from build123d import *

# Parameters (mm, degrees)
BOSS_EXTRUDE3_DEPTH = 4.5
SKETCH2_R           = 3.5
CUT_EXTRUDE2_DEPTH  = 4.5
SKETCH3_R           = 3.5
CUT_EXTRUDE3_DEPTH  = 4.5
SKETCH4_R           = 3.5
CUT_EXTRUDE4_DEPTH  = 4.5
SKETCH5_R           = 3.5
CUT_EXTRUDE5_DEPTH  = 4.5
SKETCH6_R           = 3.5
CUT_EXTRUDE6_DEPTH  = 4.5
SKETCH7_R           = 3.5
CUT_EXTRUDE7_DEPTH  = 4.5
SKETCH8_R           = 3.5
CUT_EXTRUDE8_DEPTH  = 4.5
SKETCH9_R           = 3.5
CUT_EXTRUDE9_DEPTH  = 4.5


with BuildPart() as part:
    # Sketch1 → Boss-Extrude3 (new body)
    with BuildSketch(Plane(origin=(0, 0, 0), x_dir=(1, 0, 0), z_dir=(0, 1, 0))):
        Polygon((-183.349573846, -2.857581752), (-179.118755434, 0), (-187.675629618, 0), align=None)
        Polygon((-179.118755434, 0), (-151.388696713, 0), (-165.408042798, 9.260497243), align=None)
        Polygon((-165.284400003, -14.790555769), (-147.342868955, -2.672476774), (-151.388696713, 0), (-179.118755434, 0), (-183.349573846, -2.857581752), align=None)
        Polygon((-147.342868955, -2.672476774), (-143.386109387, 0), (-151.388696713, 0), align=None)
        Polygon((-143.386109387, 0), (0, 96.845926684), (-35.732646047, 96.845926684), (-165.408042798, 9.260497243), (-151.388696713, 0), align=None)
        Polygon((-36.286932906, -100), (0, -100), (-147.342868955, -2.672476774), (-165.284400003, -14.790555769), align=None)
        Polygon((-165.408042798, 9.260497243), (-298.002482939, 96.845926684), (-319.003928208, 86.749077997), (-187.675629618, 0), (-179.118755434, 0), align=None)
        Polygon((-312.316233719, -89.964315732), (-291.442010442, -100), (-165.284400003, -14.790555769), (-183.349573846, -2.857581752), align=None)
        Polygon((0, -120), (0, -100), (-36.286932906, -100), (-291.442010442, -100), (-312.316233719, -89.964315732), (-380, -57.424043482), (-380, 0), (-400, 0), (-400, -70), (-296, -120), align=None)
        Polygon((130, -24.166666667), (0, -100), (0, -120), (150, -32.5), (150, 0), (130, 0), align=None)
        Polygon((0, 120), (0, 96.845926684), (130, 21.012593351), (130, 0), (150, 0), (150, 32.5), align=None)
        Polygon((-35.732646047, 96.845926684), (0, 96.845926684), (0, 120), (-296, 120), (-400, 70), (-400, 0), (-380, 0), (-380, 57.424043482), (-319.003928208, 86.749077997), (-298.002482939, 96.845926684), align=None)
    extrude(amount=BOSS_EXTRUDE3_DEPTH)

    # Sketch2 → Cut-Extrude2 (cut)
    with BuildSketch(Plane(origin=(0, 4.5, 0), x_dir=(1, 0, 0), z_dir=(0, 1, 0))):
        with Locations((-16.286932906, -110)):
            Circle(SKETCH2_R)
        with Locations((-36.286932906, -110)):
            Circle(SKETCH2_R)
    cut_extrude2 = extrude(amount=-CUT_EXTRUDE2_DEPTH, mode=Mode.SUBTRACT)

    # Mirror1: Cut-Extrude2 across plane
    add(cut_extrude2.mirror(Plane.XY), mode=Mode.SUBTRACT)

    # Sketch3 → Cut-Extrude3 (cut)
    with BuildSketch(Plane(origin=(0, 4.5, 0), x_dir=(1, 0, 0), z_dir=(0, 1, 0))):
        with Locations((-287.942010442, -110)):
            Circle(SKETCH3_R)
        with Locations((-267.942010442, -110)):
            Circle(SKETCH3_R)
    cut_extrude3 = extrude(amount=-CUT_EXTRUDE3_DEPTH, mode=Mode.SUBTRACT)

    # Mirror2: Cut-Extrude3 across plane
    add(cut_extrude3.mirror(Plane.XY), mode=Mode.SUBTRACT)

    # Sketch4 → Cut-Extrude4 (cut)
    with BuildSketch(Plane(origin=(0, 4.5, 0), x_dir=(1, 0, 0), z_dir=(0, 1, 0))):
        with Locations((140, 8.422963342)):
            Circle(SKETCH4_R)
        with Locations((140, -11.577036658)):
            Circle(SKETCH4_R)
    extrude(amount=-CUT_EXTRUDE4_DEPTH, mode=Mode.SUBTRACT)

    # Sketch5 → Cut-Extrude5 (cut)
    with BuildSketch(Plane(origin=(0, 4.5, 0), x_dir=(1, 0, 0), z_dir=(0, 1, 0))):
        with Locations((-390, 53.924043482)):
            Circle(SKETCH5_R)
        with Locations((-390, 33.924043482)):
            Circle(SKETCH5_R)
    cut_extrude5 = extrude(amount=-CUT_EXTRUDE5_DEPTH, mode=Mode.SUBTRACT)

    # Mirror3: Cut-Extrude5 across plane
    add(cut_extrude5.mirror(Plane.XY), mode=Mode.SUBTRACT)

    # Sketch6 → Cut-Extrude6 (cut)
    with BuildSketch(Plane(origin=(0, 4.5, 0), x_dir=(1, 0, 0), z_dir=(0, 1, 0))):
        with Locations((-237.21688879, 44.709233314)):
            Circle(SKETCH6_R)
        with Locations((-220.528931491, 33.685981472)):
            Circle(SKETCH6_R)
    extrude(amount=-CUT_EXTRUDE6_DEPTH, mode=Mode.SUBTRACT)

    # Sketch7 → Cut-Extrude7 (cut)
    with BuildSketch(Plane(origin=(0, 4.5, 0), x_dir=(1, 0, 0), z_dir=(0, 1, 0))):
        with Locations((-242.235781203, -54.69781901)):
            Circle(SKETCH7_R)
        with Locations((-225.662040668, -43.503573852)):
            Circle(SKETCH7_R)
    extrude(amount=-CUT_EXTRUDE7_DEPTH, mode=Mode.SUBTRACT)

    # Sketch8 → Cut-Extrude8 (cut)
    with BuildSketch(Plane(origin=(0, 4.5, 0), x_dir=(1, 0, 0), z_dir=(0, 1, 0))):
        with Locations((-94.973221843, 44.766341696)):
            Circle(SKETCH8_R)
        with Locations((-111.546962379, 33.572096538)):
            Circle(SKETCH8_R)
    extrude(amount=-CUT_EXTRUDE8_DEPTH, mode=Mode.SUBTRACT)

    # Sketch9 → Cut-Extrude9 (cut)
    with BuildSketch(Plane(origin=(0, 4.5, 0), x_dir=(1, 0, 0), z_dir=(0, 1, 0))):
        with Locations((-95.871017698, -48.656965194)):
            Circle(SKETCH9_R)
        with Locations((-79.183060399, -59.680217036)):
            Circle(SKETCH9_R)
    extrude(amount=-CUT_EXTRUDE9_DEPTH, mode=Mode.SUBTRACT)


solid = part.part
Part model, mm, in its own coordinate system. A direction names the side the tool comes from. Give positions to 0.01 mm unless a question says otherwise; leave off trailing zeros. Order: outer loops, then holes, each group sorted by start corner. A loop starts at its lowest first (then second) coordinate and runs counter-clockwise, first axis right, second up. Notation, with made-up numbers: (45, 26) -> (56, 26) arc R15 ccw to (56, 47) -> close; hole circle Ø8 at (78.25, 67.5). An arc over 180 degrees is marked (long way). Use one line per item in the form item = value.
(1) Flat gauge pin, fed straight in: P1, Ø4, axis at x = -242.24, z = 54.7, coming from the -Y side. Where does the tip first touch, or does it go through?
Solution:
P1 = through
(2) Saw through at A-A (z = -75.5). Write the cut outline in (x, y), then the cut area to 3 significant figures.
Solution:
outline = (-388.56, 0) -> (-342.4, 0) -> (-342.4, 4.5) -> (-388.56, 4.5) -> close; (-301.97, 0) -> (-265.69, 0) -> (-265.69, 4.5) -> (-301.97, 4.5) -> close; (-67.34, 0) -> (-31.6, 0) -> (-31.6, 4.5) -> (-67.34, 4.5) -> close; (36.59, 0) -> (76.29, 0) -> (76.29, 4.5) -> (36.59, 4.5) -> close
area = 710 mm²
(3) Saw through at B-B (x = -137.5). Write the cut outline in (y, z), then the cut area to 3 significant figures.
Solution:
outline = (0, -120) -> (4.5, -120) -> (4.5, -96.85) -> (0, -96.85) -> close; (0, -28.11) -> (4.5, -28.11) -> (4.5, -3.98) -> (0, -3.98) -> close; (0, 9.17) -> (4.5, 9.17) -> (4.5, 33.14) -> (0, 33.14) -> close; (0, 100) -> (4.5, 100) -> (4.5, 120) -> (0, 120) -> close
area = 411 mm²
(4) Drill centre lines: line 1 (X direction, y = 2.6, z = 2); line 2 (X direction, y = 0.45, z = 78.5); line 3 (X direction, y = 2.5, z = -88). Where is each one in solid material? Low to high. Write a range as from..to.
Solution:
line_1 = -400..-380, -184.65..-146.35, 130..150
line_2 = -382.32..-336.16, -295.34..-259.61, -68.84..-32.55, 36.86..71.14
line_3 = -362.56..-284.61, -48.83..-13.1, 15.16..54.86
(5) Tool access for faces 5 (the face through (-347.27, 2.22, -95.35)), 6 (the face through (-246.93, 2.22, 45.8)): list every direction of +Z, -Z, +X, -X, +Y, -Y with a clear straight run to the whole face (end or side of a thin tool).
Solution:
face_5 = -Z, -X, +Y, -Y
face_6 = +Y, -Y
(6) Pull direction Z, two halves, no side cores. Call faces 1 (the face through (-147, 4.5, -1)), 2 (the face through (-101.69, 2.22, 56.8)), 3 (the face through (-349.93, 2.22, -71.88)), 4 (the face through (73.95, 2.218, 76.862)): +Z half, -Z half, draft (parallel to the pull), parting line (faces both ways), or undercut.
Solution:
face_1 = draft
face_2 = undercut
face_3 = undercut
face_4 = +Z half
(7) Saw through at D-D (y = 2.6). Count the separate pieces of the cut face and the enclosed holes in it, then the cut area to 3 significant figures.
Solution:
separate_pieces = 1
enclosed_holes = 26
area = 39,200 mm²
(8) Saw through at C-C (x = 114.5). Write the cut outline in (y, z), then the cut area to 3 significant figures.
Solution:
outline = (0, -53.21) -> (4.5, -53.21) -> (4.5, -30.05) -> (0, -30.05) -> close; (0, 33.21) -> (4.5, 33.21) -> (4.5, 53.21) -> (0, 53.21) -> close
area = 194 mm²
